Design review of the part built by this model. Coordinates are the model's own, in mm. A direction names the side the tool comes from. Give positions to 0.01 mm unless a question says otherwise; leave off trailing zeros. Loops run counter-clockwise (first coordinate to the right, second up) from the corner with the lowest first, then second, coordinate; pieces in that order, holes last. Notation, with made-up numbers: (66, -33.75) -> (78, -33.75) arc R20 ccw to (78, -9.75) -> close; hole circle Ø6 at (20, 3.5). An arc over 180 degrees is marked (long way). Answer as CSV lines item,"result".
from build123d import *

# Parameters (mm, degrees)
EXTRUDE_1_DEPTH     = 5
SKETCH_2_R          = 12.5
SKETCH_2_R_2        = 1.5
SKETCH_2_R_3        = 4
EXTRUDE_2_DEPTH     = 5
SKETCH_3_W          = 10
SKETCH_3_H          = 5
EXTRUDE_3_DEPTH     = 5
CUT_EXTRUDE_1_DEPTH = 10


with BuildPart() as part:
    # 草图1 → 凸台-拉伸1 (new body)
    with BuildSketch(Plane(origin=(0, 0, 0), x_dir=(1, 0, 0), z_dir=(0, 1, 0))):
        with BuildLine():
            ThreePointArc((15, 11.55), (0, 26.55), (-15, 11.55))
            Line((-15, 11.55), (-12.5, 11.55))
            ThreePointArc((-12.5, 11.55), (0, 24.05), (12.5, 11.55))
            Line((12.5, 11.55), (15, 11.55))
        make_face()
        with BuildLine():
            Line((-12.5, 11.55), (-15, 11.55))
            ThreePointArc((-15, 11.55), (0, -3.45), (15, 11.55))
            Line((15, 11.55), (12.5, 11.55))
            ThreePointArc((12.5, 11.55), (0, -0.95), (-12.5, 11.55))
        make_face()
        with BuildLine():
            ThreePointArc((15, 11.55), (0, 26.55), (-15, 11.55))
            Line((-15, 11.55), (-12.5, 11.55))
            ThreePointArc((-12.5, 11.55), (0, 24.05), (12.5, 11.55))
            Line((12.5, 11.55), (15, 11.55))
        make_face()
        with BuildLine():
            Line((-12.5, 11.55), (-15, 11.55))
            ThreePointArc((-15, 11.55), (0, -3.45), (15, 11.55))
            Line((15, 11.55), (12.5, 11.55))
            ThreePointArc((12.5, 11.55), (0, -0.95), (-12.5, 11.55))
        make_face()
        with BuildLine():
            Line((-15, 11.55), (-15, -11.55))
            Line((-15, -11.55), (15, -11.55))
            Line((15, -11.55), (15, 11.55))
            ThreePointArc((15, 11.55), (0, -3.45), (-15, 11.55))
        make_face()
    extrude(amount=EXTRUDE_1_DEPTH)

    # 草图2 → 凸台-拉伸2 (add)
    with BuildSketch(Plane(origin=(0, 5, 0), x_dir=(1, 0, 0), z_dir=(0, 1, 0))):
        with Locations((0, 11.55)):
            Circle(SKETCH_2_R)
        with Locations((-8.5, 11.55)):
            Circle(SKETCH_2_R_2, mode=Mode.SUBTRACT)
        with Locations((8.5, 11.55)):
            Circle(SKETCH_2_R_2, mode=Mode.SUBTRACT)
        with Locations((0, 11.55)):
            Circle(SKETCH_2_R_3, mode=Mode.SUBTRACT)
    extrude(amount=-EXTRUDE_2_DEPTH)

    # 草图3 → 凸台-拉伸3 (add)
    with BuildSketch(Plane(origin=(0, 5, 0), x_dir=(1, 0, 0), z_dir=(0, 1, 0))):
        with Locations((0, -14.05)):
            Rectangle(SKETCH_3_W, SKETCH_3_H)
    extrude(amount=-EXTRUDE_3_DEPTH)

    # 草图4 → 切除-拉伸1 (cut)
    with BuildSketch(Plane(origin=(0, 5, 0), x_dir=(1, 0, 0), z_dir=(0, 1, 0))):
        with BuildLine():
            ThreePointArc((15, 11.55), (0, 26.55), (-15, 11.55))
            Line((-15, 11.55), (-12.5, 11.55))
            ThreePointArc((-12.5, 11.55), (0, 24.05), (12.5, 11.55))
            Line((12.5, 11.55), (15, 11.55))
        make_face()
        with BuildLine():
            ThreePointArc((12.5, 11.55), (0, 24.05), (-12.5, 11.55))
            Line((-12.5, 11.55), (-10, 11.55))
            ThreePointArc((-10, 11.55), (-8.5, 13.05), (-7, 11.55))
            Line((-7, 11.55), (-4, 11.55))
            ThreePointArc((-4, 11.55), (0, 15.55), (4, 11.55))
            Line((4, 11.55), (7, 11.55))
            ThreePointArc((7, 11.55), (8.5, 13.05), (10, 11.55))
            Line((10, 11.55), (12.5, 11.55))
        make_face()
        with BuildLine():
            Line((-10, 11.55), (-12.5, 11.55))
            ThreePointArc((-12.5, 11.55), (0, -0.95), (12.5, 11.55))
            Line((12.5, 11.55), (10, 11.55))
            ThreePointArc((10, 11.55), (8.5, 10.05), (7, 11.55))
            Line((7, 11.55), (4, 11.55))
            ThreePointArc((4, 11.55), (0, 7.55), (-4, 11.55))
            Line((-4, 11.55), (-7, 11.55))
            ThreePointArc((-7, 11.55), (-8.5, 10.05), (-10, 11.55))
        make_face()
        with BuildLine():
            ThreePointArc((12.5, 11.55), (0, 24.05), (-12.5, 11.55))
            Line((-12.5, 11.55), (-10, 11.55))
            ThreePointArc((-10, 11.55), (-8.5, 13.05), (-7, 11.55))
            Line((-7, 11.55), (-4, 11.55))
            ThreePointArc((-4, 11.55), (0, 15.55), (4, 11.55))
            Line((4, 11.55), (7, 11.55))
            ThreePointArc((7, 11.55), (8.5, 13.05), (10, 11.55))
            Line((10, 11.55), (12.5, 11.55))
        make_face()
        with BuildLine():
            Line((-10, 11.55), (-12.5, 11.55))
            ThreePointArc((-12.5, 11.55), (0, -0.95), (12.5, 11.55))
            Line((12.5, 11.55), (10, 11.55))
            ThreePointArc((10, 11.55), (8.5, 10.05), (7, 11.55))
            Line((7, 11.55), (4, 11.55))
            ThreePointArc((4, 11.55), (0, 7.55), (-4, 11.55))
            Line((-4, 11.55), (-7, 11.55))
            ThreePointArc((-7, 11.55), (-8.5, 10.05), (-10, 11.55))
        make_face()
    extrude(amount=-CUT_EXTRUDE_1_DEPTH, mode=Mode.SUBTRACT)


solid = part.part
Q1. We need section C-C, the plane x = 0.5. State the section outline as (y, z) points, and give its area (4 significant figures).
Filled sheet:
outline,"(0, 0.94) -> (5, 0.94) -> (5, 16.55) -> (0, 16.55) -> close"
area,"78.05 mm^2"
Q2. The part is to be moulded in two halves that separate along X. For faces 4 (the flat face through (15, 2, 0)), 5 (the flat face through (-15, 2, 0)), 6 (the flat face through (-14, 3, -11.55)), 7 (the cylindrical face through (-0.275, 2.535, 0.947)), say which applies: pulls with the +X half, pulls with the -X half, needs draft (parallel to the pull), parting line crosses it, or undercut.
Filled sheet:
face 4,"pulls with the +X half"
face 5,"pulls with the -X half"
face 6,"needs draft"
face 7,"undercut"
Q3. Clearance check with flat-ended pins moving along their axes: pin 1 Ø1 at (y, z) = (2.5, 13.5) entering from -X; pin 2 Ø5 at (x, z) = (1.5, 12) entering from -Y. State where each tip first meets the part, or that it passes through.
Filled sheet:
pin 1,"stops at x = -5"
pin 2,"stops at y = 0"
Q4. We need section A-A, the plane y = 4.25. State the section outline as (x, z) points.
Filled sheet:
outline,"(-15, -11.55) -> (-12.5, -11.55) arc R12.5 cw to (12.5, -11.55) -> (15, -11.55) -> (15, 11.55) -> (5, 11.55) -> (5, 16.55) -> (-5, 16.55) -> (-5, 11.55) -> (-15, 11.55) -> close"
Q5. To check wall thickness, follow probe 1 along X at (y, z) = (4.7, 13.75); probe 2 along X at (y, z) = (4.8, -0.75); probe 3 along X at (y, z) = (3.45, -2.75). State the ranges of each line that lie inside material, in increasing order. Write a range as from..to.
Filled sheet:
probe 1,"x = -5..5"
probe 2,"x = -15..-6.29, 6.29..15"
probe 3,"x = -15..-8.88, 8.88..15"
Q6. We need section D-D, the plane z = 13.25. State the section outline as (x, y) points.
Filled sheet:
outline,"(-5, 0) -> (5, 0) -> (5, 5) -> (-5, 5) -> close"
Q7. For faces 1 (the flat face through (5, 3, 14)), 2 (the flat face through (-5, 3, 14)), 3 (the flat face through (14, 3, -11.55)), list the 3-axis set-ups (+Z, -Z, +X, -X, +Y, -Y) from which the entire face can be reached by the end or side of a thin tool; tool diameter is ignored.
Filled sheet:
face 1,"+Z, +X, +Y, -Y"
face 2,"+Z, -X, +Y, -Y"
face 3,"-Z, +X, -X, +Y, -Y"
Q8. We need section B-B, the plane z = -8.25. State the section outline as (x, y) points.
Filled sheet:
outline,"(-15, 0) -> (-12.06, 0) -> (-12.06, 5) -> (-15, 5) -> close; (12.06, 0) -> (15, 0) -> (15, 5) -> (12.06, 5) -> close"
